Geometry: final body of the model. Coordinates: model frame, mm. A direction names the side the tool comes from. Coordinates: 2 decimals unless noted, no trailing zeros. Order: outer loops, then holes, each group sorted by start corner. A loop starts at its lowest first (then second) coordinate and runs counter-clockwise, first axis right, second up. Notation, with made-up numbers: (32, -26.5) -> (37, -26.5) arc R19 cw to (37, 2.5) -> close; hole circle Ø4 at (14, -20). An arc over 180 degrees is marked (long way). Use CSV: the item, a comma, the result in double quotes. Start each with the question number.
from build123d import *

# Parameters (mm, degrees)
EXTRUDE_DEPTH = 50


with BuildPart() as part:
    # Sketch → Extrude (new body)
    with BuildSketch(Plane.XY):
        with BuildLine():
            Line((-42, 60), (42, 60))
            ThreePointArc((60, 42), (54.727922, 54.727922), (42, 60))
            Line((60, 42), (60, -42))
            ThreePointArc((42, -60), (54.727922, -54.727922), (60, -42))
            Line((42, -60), (-42, -60))
            ThreePointArc((-60, -42), (-54.727922, -54.727922), (-42, -60))
            Line((-60, -42), (-60, 42))
            ThreePointArc((-42, 60), (-54.727922, 54.727922), (-60, 42))
        make_face()
        with BuildLine():
            Line((-36, 48), (36, 48))
            ThreePointArc((48, 36), (44.485281, 44.485281), (36, 48))
            Line((48, 36), (48, -36))
            ThreePointArc((36, -48), (44.485281, -44.485281), (48, -36))
            Line((36, -48), (-36, -48))
            ThreePointArc((-48, -36), (-44.485281, -44.485281), (-36, -48))
            Line((-48, -36), (-48, 36))
            ThreePointArc((-36, 48), (-44.485281, 44.485281), (-48, 36))
        make_face(mode=Mode.SUBTRACT)
    extrude(amount=EXTRUDE_DEPTH)


solid = part.part
(1) Section D-D (x = -51). Return loops of the section in (y, z), then the cut area to 3 significant figures.
(2) Mould query, pull axis Y, two halves, no side actions, for faces 1 (the face through (54.587, -54.867, 24.65)), 2 (the face through (-1, 48, 25)), 3 (the face through (-60, -1, 25)). Classes: pulls with the +Y half, pulls with the -Y half, needs draft (parallel to the pull), parting line crosses it, or undercut.
(3) Section B-B (z = 8). Return loops of the section in (x, y).
(4) Section A-A (x = -24). Return loops of the section in (y, z), then the cut area to 3 significant figures.
(5) Line query: line 1 (Y direction, x = -12, z = 29); line 2 (X direction, y = 39, z = 5.5). Output: solid intervals per line, ascending. Write a range as from..to.
(6) Access query for faces 4 (the face through (1, -60, 25)), 5 (the face through (-44.39, 44.58, 24.65)). Directions: +Z, -Z, +X, -X, +Y, -Y. A direction counts if a zero-diameter tool reaches every point of the face in a straight line with its end or side. Return the directions, or none.
Check sheet entries:
1,outline,"(-57.59, 0) -> (57.59, 0) -> (57.59, 50) -> (-57.59, 50) -> close"
1,area,"5,760 mm^2"
2,face 1,"pulls with the -Y half"
2,face 2,"undercut"
2,face 3,"needs draft"
3,outline,"(-60, -42) arc R18 ccw to (-42, -60) -> (42, -60) arc R18 ccw to (60, -42) -> (60, 42) arc R18 ccw to (42, 60) -> (-42, 60) arc R18 ccw to (-60, 42) -> close; hole (-48, -36) arc R12 ccw to (-36, -48) -> (36, -48) arc R12 ccw to (48, -36) -> (48, 36) arc R12 ccw to (36, 48) -> (-36, 48) arc R12 ccw to (-48, 36) -> close"
4,outline,"(-60, 0) -> (-48, 0) -> (-48, 50) -> (-60, 50) -> close; (48, 0) -> (60, 0) -> (60, 50) -> (48, 50) -> close"
4,area,"1,200 mm^2"
5,line 1,"y = -60..-48, 48..60"
5,line 2,"x = -60..-47.62, 47.62..60"
6,face 4,"+Z, -Z, +X, -X, -Y"
6,face 5,"+Z, -Z"
